The model under review builds one solid part; all positions refer to its coordinate system, in mm. Give positions to 0.01 mm unless a question says otherwise; leave off trailing zeros. Order: outer loops, then holes, each group sorted by start corner. A loop starts at its lowest first (then second) coordinate and runs counter-clockwise, first axis right, second up. Notation, with made-up numbers: (11.5, -10.5) - (45.5, -10.5) arc R27 cw to (45.5, 10.5) - close; hole circle Ø11 at (-25.5, -39.75). An arc over 180 degrees is marked (long way). Use CSV: the item, a comma, the result in double quotes. Start each with the question number.
1. For pin 1 (6 mm diameter, centred on x = 96.24, y = 6.35, fed in from +Z); pin 2 (1.5 mm diameter, centred on x = 82.5, z = -102, fed in from -Y), all flat-tipped, find the tip position at first contact; note any pin that passes through.
2. Take a section at C-C, the plane x = 117. State the section outline as (y, z) points.
3. To check wall thickness, follow line 1 (X direction, y = 6.5, z = -99.75); line 2 (X direction, y = 10.25, z = -104.75); line 3 (X direction, y = 12.25, z = -106). State the ranges of each line that lie inside material, in increasing order. Write a range as [from, to].
4. Take a section at D-D, the plane x = 94. State the section outline as (y, z) points.
5. Draft analysis for pull direction Z (two halves, no side actions). For faces 1 (the flat face through (96, 12, -98.821)), 2 (the flat face through (96, 12, -111.521)), 3 (the cylindrical face through (76.223, 6.439, -105.431)), 4 (the cylindrical face through (91.245, 6.57, -105.082)), state which applies: released by +Z, released by -Z, zero draft, split by the parting line, or undercut.
6. Take a section at A-A, the plane z = -105.75. State the section outline as (x, y) points.
7. Take a section at B-B, the plane y = 6.35. State the section outline as (x, z) points, then the cut area to 3 significant figures.
```python
from build123d import *

# Parameters (mm, degrees)
SKETCH1_W           = 75
SKETCH1_H           = 12.7
BOSS_EXTRUDE2_DEPTH = 12.7
SKETCH2_R           = 2
CUT_EXTRUDE1_DEPTH  = 175.598479387
SKETCH3_R           = 5
CUT_EXTRUDE2_DEPTH  = 135.940675175


with BuildPart() as part:
    # Sketch1 → Boss-Extrude2 (new body)
    with BuildSketch(Plane(origin=(0, 0, 0), x_dir=(1, 0, 0), z_dir=(0, 1, 0))):
        with Locations((96.240068104, 105.170998865)):
            Rectangle(SKETCH1_W, SKETCH1_H)
    extrude(amount=BOSS_EXTRUDE2_DEPTH)

    # Sketch2 → Cut-Extrude1 (cut, through all)
    with BuildSketch(Plane(origin=(0, 12.7, 0), x_dir=(1, 0, 0), z_dir=(0, 1, 0))):
        with Locations(Location((74.240068104, 105.170998865, 0), (0, 0, 270))):
            Circle(SKETCH2_R)
        with Locations(Location((64.240068104, 105.170998865, 0), (0, 0, 270))):
            Circle(SKETCH2_R)
        with Locations(Location((118.240068104, 105.170998865, 0), (0, 0, 270))):
            Circle(SKETCH2_R)
        with Locations(Location((128.240068104, 105.170998865, 0), (0, 0, 270))):
            Circle(SKETCH2_R)
    extrude(amount=-CUT_EXTRUDE1_DEPTH, mode=Mode.SUBTRACT)

    # Sketch3 → Cut-Extrude2 (cut, through all)
    with BuildSketch(Plane.XY.offset(-98.820998865)):
        with Locations((96.240068104, 6.35)):
            Circle(SKETCH3_R)
    extrude(amount=-CUT_EXTRUDE2_DEPTH, mode=Mode.SUBTRACT)


solid = part.part
```
Determined:
1,pin 1,"passes through"
1,pin 2,"stops at y = 0"
2,outline,"(0, -111.52) - (12.7, -111.52) - (12.7, -106.74) - (0, -106.74) - close; (0, -103.6) - (12.7, -103.6) - (12.7, -98.82) - (0, -98.82) - close"
3,line 1,"x = [58.74, 91.24], [101.24, 133.74]"
3,line 2,"x = [58.74, 62.28], [66.2, 72.28], [76.2, 93.11], [99.37, 116.28], [120.2, 126.28], [130.2, 133.74]"
3,line 3,"x = [58.74, 62.42], [66.06, 72.42], [76.06, 116.42], [120.06, 126.42], [130.06, 133.74]"
4,outline,"(0, -111.52) - (1.88, -111.52) - (1.88, -98.82) - (0, -98.82) - close; (10.82, -111.52) - (12.7, -111.52) - (12.7, -98.82) - (10.82, -98.82) - close"
5,face 1,"released by +Z"
5,face 2,"released by -Z"
5,face 3,"undercut"
5,face 4,"zero draft"
6,outline,"(58.74, 0) - (62.33, 0) - (62.33, 12.7) - (58.74, 12.7) - close; (66.15, 0) - (72.33, 0) - (72.33, 12.7) - (66.15, 12.7) - close; (76.15, 0) - (116.33, 0) - (116.33, 12.7) - (76.15, 12.7) - close; (120.15, 0) - (126.33, 0) - (126.33, 12.7) - (120.15, 12.7) - close; (130.15, 0) - (133.74, 0) - (133.74, 12.7) - (130.15, 12.7) - close; hole circle Ø10 at (96.24, 6.35)"
7,outline,"(58.74, -111.52) - (91.24, -111.52) - (91.24, -98.82) - (58.74, -98.82) - close; (101.24, -111.52) - (133.74, -111.52) - (133.74, -98.82) - (101.24, -98.82) - close; hole circle Ø4 at (64.24, -105.17); hole circle Ø4 at (74.24, -105.17); hole circle Ø4 at (118.24, -105.17); hole circle Ø4 at (128.24, -105.17)"
7,area,"775 mm²"
